Input: part model. Units: mm. Frame: model coordinates. A direction names the side the tool comes from. Give positions to 0.01 mm unless a question says otherwise; leave off trailing zeros. Write each loop counter-clockwise with the first axis right and the second up, starting at its lowest first coordinate (ties: lowest second). Pieces come first, ordered by that corner, then holes.
Autodesk Inventor part; units mm, degrees
ref_plane "IP1_XY" through (0, 0, 0) normal (1, 0, 0) x (0, 0, -1)
ref_plane "IP1_YZ" through (0, 0, 0) normal (0, 0, -1) x (0, 1, 0)
ref_plane "IP1_ZX" through (0, 0, 0) normal (0, 1, 0) x (1, 0, 0)
sketch "Sketch_1" plane through (0, 0, 0) normal (0, 1, 0) x (-1, 0, 0)
  line L0 (-6, 0) -> (2.61, 0)
  line L1 (0.8226, 0) -> (1.4, -1)
  line L2 (1.4, -1) -> (2.46, -1)
  line L3 (2.46, -1) -> (2.61, -1.15)
  line L4 (2.61, -1.15) -> (2.61, -2)
  arc A0 (2.36, -2.25) -> (2.61, -2) centre (2.36, -2) ccw
  line L5 (2.36, -2.25) -> (0, -2.25)
  line L6 (0, -2.25) -> (0, -1.55)
  arc A1 (0, -1.55) -> (-0.0656, -1.4561) centre (-0.1, -1.55) ccw
  line L7 (-0.0656, -1.4561) -> (-0.4756, -1.3061)
  arc A2 (-0.4756, -1.3061) -> (-0.51, -1.3) centre (-0.51, -1.4) ccw
  line L8 (-0.51, -1.3) -> (-5.724, -1.3)
  line L9 (-5.724, -1.3) -> (-6, -1.024)
  line L10 (-6, -1.024) -> (-6, 0)
  line L11 (-6, 0) -> (0.8226, 0)
revolve "Revolution1" add sketch "Sketch_1" angle 360 about axis through (6, 0, 0) along (1, 0, 0)
thread "Thread1"
sketch "Skizze_1" plane through (-1.4, 0, 0) normal (1, 0, 0) x (0, 0, -1)
  line L0 (-1, -0.5774) -> (0, -1.1547)
  line L1 (0, -1.1547) -> (1, -0.5774)
  line L2 (1, -0.5774) -> (1, 0.5774)
  line L3 (1, 0.5774) -> (0, 1.1547)
  line L4 (0, 1.1547) -> (-1, 0.5774)
  line L5 (-1, 0.5774) -> (-1, -0.5774)
extrude "Extrusion1" cut sketch "Skizze_1" against normal blind 2.2
ref_plane "IP1_XY" through (0, 0, 0) normal (1, 0, 0) x (0, 0, -1)
ref_plane "IP1_YZ" through (0, 0, 0) normal (0, 0, -1) x (0, 1, 0)
ref_plane "IP1_ZX" through (0, 0, 0) normal (0, 1, 0) x (1, 0, 0)
ref_plane "IP2_XY" through (-2.6, 0, 0) normal (1, 0, 0) x (0, 0, -1)
ref_plane "IP2_YZ" through (-2.6, 0, 0) normal (0, 0, -1) x (0, 1, 0)
ref_plane "IP2_ZX" through (-2.6, 0, 0) normal (0, 1, 0) x (1, 0, 0)
ref_plane "IP3_XY" through (6, 0, 0) normal (1, 0, 0) x (0, 0, -1)
ref_plane "IP3_YZ" through (6, 0, 0) normal (0, 0, -1) x (0, 1, 0)
ref_plane "IP3_ZX" through (6, 0, 0) normal (0, 1, 0) x (1, 0, 0)
ref_plane "IP4_XY" through (0, 0, 0) normal (1, 0, 0) x (0, 0, -1)
ref_plane "IP4_YZ" through (0, 0, 0) normal (0, 0, -1) x (0, 1, 0)
ref_plane "IP4_ZX" through (0, 0, 0) normal (0, 1, 0) x (1, 0, 0)
properties part number "M2.6x66"
Q1. Pin query (flat end, axial travel): pin 1 (1.5 mm diameter, centred on x = 0.5, y = -0.5, fed in from -Z); pin 2 (0.6 mm diameter, centred on y = -0.5, z = 0, fed in from -X). Return the tip coordinate at first contact, or that it passes through.
Q2. Section B-B, the plane x = -0.25. Return the cut outline in (y, z).
Q3. Material intervals for line 1 along X through (y, z) = (1.6, 0); line 2 along Z through (x, y) = (-2, 0.3); line 3 along Z through (x, y) = (-1.5, -1.6), sorted ascending.
Q4. Access query for faces 1 (the cylindrical face through (-1.16, 2.23, 0.29)), 2 (the flat face through (-2, -0.86, 0.51)), 3 (the flat face through (0, 0, 2)). Directions: +Z, -Z, +X, -X, +Y, -Y. A direction counts if a zero-diameter tool reaches every point of the face in a straight line with its end or side. Return the directions, or none.
Q5. Section A-A, the plane x = 1.5. Return the cut outline in (y, z).
Q6. Mould query, pull axis Y, two halves, no side actions, for faces 4 (the flat face through (-2.61, -1, -1)), 5 (the cylindrical face through (3.15, 1.29, 0.17)), 6 (the flat face through (-2, 0, -1)). Classes: +Y half, -Y half, draft (parallel to the pull), parting line (faces both ways), or undercut.
Solutions:
1. pin 1: stops at z = -2.25
1. pin 2: stops at x = -1.28
2. outline: circle Ø4.5 at (0, 0)
3. line 1: x = -2.61 to 0
3. line 2: z = -2.23 to -1, 1 to 2.23
3. line 3: z = -1.58 to 1.58
4. face 1: +X, -X
4. face 2: -X
4. face 3: +X
5. outline: circle Ø2.6 at (0, 0)
6. face 4: draft
6. face 5: parting line
6. face 6: undercut
